```python
from build123d import *

# Parameters (mm, degrees)
F0_W     = 39.85
F0_H     = 7.85
F1_DEPTH = 3


with BuildPart() as f1:
    # F0 (on Top) → F1 (new body)
    with BuildSketch(Plane.XY):
        Rectangle(F0_W, F0_H)
        with BuildLine():
            ThreePointArc((-16.8, 2.1830311496), (-16, 2.325), (-15.2, 2.1830311496))
            Line((-15.2, 2.1830311496), (-15.2, 1.1))
            ThreePointArc((-15.2, 1.1), (-15.1121320344, 0.8878679656), (-14.9, 0.8))
            Line((-14.9, 0.8), (-13.8169688504, 0.8))
            ThreePointArc((-13.8169688504, 0.8), (-13.675, 0), (-13.8169688504, -0.8))
            Line((-13.8169688504, -0.8), (-14.9, -0.8))
            ThreePointArc((-14.9, -0.8), (-15.1121320344, -0.8878679656), (-15.2, -1.1))
            Line((-15.2, -1.1), (-15.2, -2.1830311496))
            ThreePointArc((-15.2, -2.1830311496), (-16, -2.325), (-16.8, -2.1830311496))
            Line((-16.8, -2.1830311496), (-16.8, -1.1))
            ThreePointArc((-16.8, -1.1), (-16.8878679656, -0.8878679656), (-17.1, -0.8))
            Line((-17.1, -0.8), (-18.1830311496, -0.8))
            ThreePointArc((-18.1830311496, -0.8), (-18.325, 0), (-18.1830311496, 0.8))
            Line((-18.1830311496, 0.8), (-17.1, 0.8))
            ThreePointArc((-17.1, 0.8), (-16.8878679656, 0.8878679656), (-16.8, 1.1))
            Line((-16.8, 1.1), (-16.8, 2.1830311496))
        make_face(mode=Mode.SUBTRACT)
        with BuildLine():
            ThreePointArc((-8.8, 2.1830311496), (-8, 2.325), (-7.2, 2.1830311496))
            Line((-7.2, 2.1830311496), (-7.2, 1.1))
            ThreePointArc((-7.2, 1.1), (-7.1121320344, 0.8878679656), (-6.9, 0.8))
            Line((-6.9, 0.8), (-5.8169688504, 0.8))
            ThreePointArc((-5.8169688504, 0.8), (-5.675, 0), (-5.8169688504, -0.8))
            Line((-5.8169688504, -0.8), (-6.9, -0.8))
            ThreePointArc((-6.9, -0.8), (-7.1121320344, -0.8878679656), (-7.2, -1.1))
            Line((-7.2, -1.1), (-7.2, -2.1830311496))
            ThreePointArc((-7.2, -2.1830311496), (-8, -2.325), (-8.8, -2.1830311496))
            Line((-8.8, -2.1830311496), (-8.8, -1.1))
            ThreePointArc((-8.8, -1.1), (-8.8878679656, -0.8878679656), (-9.1, -0.8))
            Line((-9.1, -0.8), (-10.1830311496, -0.8))
            ThreePointArc((-10.1830311496, -0.8), (-10.325, 0), (-10.1830311496, 0.8))
            Line((-10.1830311496, 0.8), (-9.1, 0.8))
            ThreePointArc((-9.1, 0.8), (-8.8878679656, 0.8878679656), (-8.8, 1.1))
            Line((-8.8, 1.1), (-8.8, 2.1830311496))
        make_face(mode=Mode.SUBTRACT)
        with BuildLine():
            ThreePointArc((-0.8, 2.1830311496), (0, 2.325), (0.8, 2.1830311496))
            Line((0.8, 2.1830311496), (0.8, 1.1))
            ThreePointArc((0.8, 1.1), (0.8878679656, 0.8878679656), (1.1, 0.8))
            Line((1.1, 0.8), (2.1830311496, 0.8))
            ThreePointArc((2.1830311496, 0.8), (2.325, 0), (2.1830311496, -0.8))
            Line((2.1830311496, -0.8), (1.1, -0.8))
            ThreePointArc((1.1, -0.8), (0.8878679656, -0.8878679656), (0.8, -1.1))
            Line((0.8, -1.1), (0.8, -2.1830311496))
            ThreePointArc((0.8, -2.1830311496), (0, -2.325), (-0.8, -2.1830311496))
            Line((-0.8, -2.1830311496), (-0.8, -1.1))
            ThreePointArc((-0.8, -1.1), (-0.8878679656, -0.8878679656), (-1.1, -0.8))
            Line((-1.1, -0.8), (-2.1830311496, -0.8))
            ThreePointArc((-2.1830311496, -0.8), (-2.325, 0), (-2.1830311496, 0.8))
            Line((-2.1830311496, 0.8), (-1.1, 0.8))
            ThreePointArc((-1.1, 0.8), (-0.8878679656, 0.8878679656), (-0.8, 1.1))
            Line((-0.8, 1.1), (-0.8, 2.1830311496))
        make_face(mode=Mode.SUBTRACT)
        with BuildLine():
            ThreePointArc((7.2, 2.1830311496), (8, 2.325), (8.8, 2.1830311496))
            Line((8.8, 2.1830311496), (8.8, 1.1))
            ThreePointArc((8.8, 1.1), (8.8878679656, 0.8878679656), (9.1, 0.8))
            Line((9.1, 0.8), (10.1830311496, 0.8))
            ThreePointArc((10.1830311496, 0.8), (10.325, 0), (10.1830311496, -0.8))
            Line((10.1830311496, -0.8), (9.1, -0.8))
            ThreePointArc((9.1, -0.8), (8.8878679656, -0.8878679656), (8.8, -1.1))
            Line((8.8, -1.1), (8.8, -2.1830311496))
            ThreePointArc((8.8, -2.1830311496), (8, -2.325), (7.2, -2.1830311496))
            Line((7.2, -2.1830311496), (7.2, -1.1))
            ThreePointArc((7.2, -1.1), (7.1121320344, -0.8878679656), (6.9, -0.8))
            Line((6.9, -0.8), (5.8169688504, -0.8))
            ThreePointArc((5.8169688504, -0.8), (5.675, 0), (5.8169688504, 0.8))
            Line((5.8169688504, 0.8), (6.9, 0.8))
            ThreePointArc((6.9, 0.8), (7.1121320344, 0.8878679656), (7.2, 1.1))
            Line((7.2, 1.1), (7.2, 2.1830311496))
        make_face(mode=Mode.SUBTRACT)
        with BuildLine():
            ThreePointArc((15.2, 2.1830311496), (16, 2.325), (16.8, 2.1830311496))
            Line((16.8, 2.1830311496), (16.8, 1.1))
            ThreePointArc((16.8, 1.1), (16.8878679656, 0.8878679656), (17.1, 0.8))
            Line((17.1, 0.8), (18.1830311496, 0.8))
            ThreePointArc((18.1830311496, 0.8), (18.325, 0), (18.1830311496, -0.8))
            Line((18.1830311496, -0.8), (17.1, -0.8))
            ThreePointArc((17.1, -0.8), (16.8878679656, -0.8878679656), (16.8, -1.1))
            Line((16.8, -1.1), (16.8, -2.1830311496))
            ThreePointArc((16.8, -2.1830311496), (16, -2.325), (15.2, -2.1830311496))
            Line((15.2, -2.1830311496), (15.2, -1.1))
            ThreePointArc((15.2, -1.1), (15.1121320344, -0.8878679656), (14.9, -0.8))
            Line((14.9, -0.8), (13.8169688504, -0.8))
            ThreePointArc((13.8169688504, -0.8), (13.675, 0), (13.8169688504, 0.8))
            Line((13.8169688504, 0.8), (14.9, 0.8))
            ThreePointArc((14.9, 0.8), (15.1121320344, 0.8878679656), (15.2, 1.1))
            Line((15.2, 1.1), (15.2, 2.1830311496))
        make_face(mode=Mode.SUBTRACT)
        with BuildLine():
            Line((-15.2, 1.1), (-15.2, 2.1830311496))
            ThreePointArc((-15.2, 2.1830311496), (-16, 2.325), (-16.8, 2.1830311496))
            Line((-16.8, 2.1830311496), (-16.8, 1.1))
            ThreePointArc((-16.8, 1.1), (-16.8878679656, 0.8878679656), (-17.1, 0.8))
            Line((-17.1, 0.8), (-18.1830311496, 0.8))
            ThreePointArc((-18.1830311496, 0.8), (-18.325, 0), (-18.1830311496, -0.8))
            Line((-18.1830311496, -0.8), (-17.1, -0.8))
            ThreePointArc((-17.1, -0.8), (-16.8878679656, -0.8878679656), (-16.8, -1.1))
            Line((-16.8, -1.1), (-16.8, -2.1830311496))
            ThreePointArc((-16.8, -2.1830311496), (-16, -2.325), (-15.2, -2.1830311496))
            Line((-15.2, -2.1830311496), (-15.2, -1.1))
            ThreePointArc((-15.2, -1.1), (-15.1121320344, -0.8878679656), (-14.9, -0.8))
            Line((-14.9, -0.8), (-13.8169688504, -0.8))
            ThreePointArc((-13.8169688504, -0.8), (-13.675, 0), (-13.8169688504, 0.8))
            Line((-13.8169688504, 0.8), (-14.9, 0.8))
            ThreePointArc((-14.9, 0.8), (-15.1121320344, 0.8878679656), (-15.2, 1.1))
        make_face()
        with BuildLine():
            Line((16.8, 1.1), (16.8, 2.1830311496))
            ThreePointArc((16.8, 2.1830311496), (16, 2.325), (15.2, 2.1830311496))
            Line((15.2, 2.1830311496), (15.2, 1.1))
            ThreePointArc((15.2, 1.1), (15.1121320344, 0.8878679656), (14.9, 0.8))
            Line((14.9, 0.8), (13.8169688504, 0.8))
            ThreePointArc((13.8169688504, 0.8), (13.675, 0), (13.8169688504, -0.8))
            Line((13.8169688504, -0.8), (14.9, -0.8))
            ThreePointArc((14.9, -0.8), (15.1121320344, -0.8878679656), (15.2, -1.1))
            Line((15.2, -1.1), (15.2, -2.1830311496))
            ThreePointArc((15.2, -2.1830311496), (16, -2.325), (16.8, -2.1830311496))
            Line((16.8, -2.1830311496), (16.8, -1.1))
            ThreePointArc((16.8, -1.1), (16.8878679656, -0.8878679656), (17.1, -0.8))
            Line((17.1, -0.8), (18.1830311496, -0.8))
            ThreePointArc((18.1830311496, -0.8), (18.325, 0), (18.1830311496, 0.8))
            Line((18.1830311496, 0.8), (17.1, 0.8))
            ThreePointArc((17.1, 0.8), (16.8878679656, 0.8878679656), (16.8, 1.1))
        make_face()
    extrude(amount=F1_DEPTH)


solid = f1.part
```
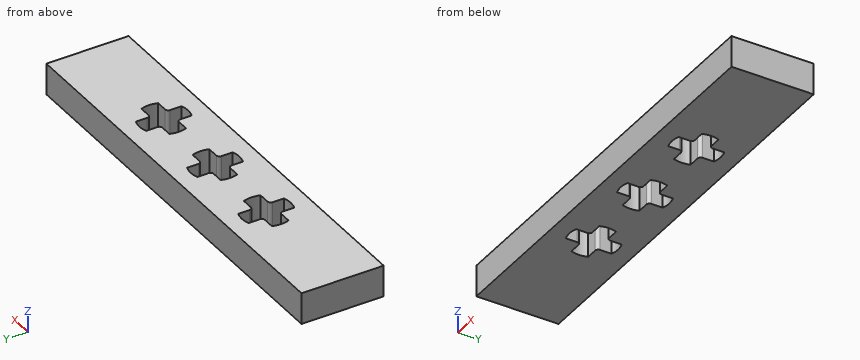
Geometry check sheet. Reference: the model listing, model coordinates, mm. Round coordinates to 2 decimals unless told otherwise and drop trailing zeros. Loops run counter-clockwise (first coordinate to the right, second up) from the corner with the lowest first, then second, coordinate; pieces in that order, holes last. Notation, with made-up numbers: M -17.5,-30.75 L 10.5,-30.75 A16 ccw 10.5,-1.75 Z; hole C 80,49 d6. An arc over 180 degrees is marked long. Return JSON: item names as keys, results as strings. Group by question number.
(1) Scan lines: line 1 along X through (y, z) = (-1.75, 1.35) (3 decimals); line 2 along X through (y, z) = (0.5, 0.5) (3 decimals); line 3 along Y through (x, z) = (6, 0.25) (3 decimals). Record each from-to range of solid material in increasing order. Write a range as [from, to].
(2) Section check A-A, the plane y = -0.25. Enter the section's corners in (x, z) (3 decimals), and give its area (3 significant figures).
(3) Section check B-B, the plane z = 0.7. Give the number of separate pieces and of enclosed holes in the cut face, and give its area (3 significant figures).
Data:
{
 "1": {"line 1": "[-19.925, -8.8], [-7.2, -0.8], [0.8, 7.2], [8.8, 19.925]", "line 2": "[-19.925, -10.271], [-5.729, -2.271], [2.271, 5.729], [10.271, 19.925]", "line 3": "[-3.925, -0.8], [0.8, 3.925]"},
 "2": {"outline": "M -19.925,0 L -10.312,0 L -10.312,3 L -19.925,3 Z; M -5.688,0 L -2.312,0 L -2.312,3 L -5.688,3 Z; M 2.312,0 L 5.688,0 L 5.688,3 L 2.312,3 Z; M 10.312,0 L 19.925,0 L 19.925,3 L 10.312,3 Z", "area": "77.9 mm²"},
 "3": {"separate pieces": "1", "enclosed holes": "3", "area": "277 mm²"}
}
